Build history of the part. All positions in model axes, mm. Face numbers are marked on the shaded views. A direction names the side the tool comes from. Coordinates: 2 decimals unless noted, no trailing zeros. Loops run counter-clockwise (first coordinate to the right, second up) from the corner with the lowest first, then second, coordinate; pieces in that order, holes last.
Item 1: Drill centre lines: line 1 along Y through (x, z) = (23, 0.6); line 2 along X through (y, z) = (1.25, 0.5); line 3 along Z through (x, y) = (6, 6.5). Where is each one in solid material? Low to high.
Item 2: Cut at B-B (x = 12.5). List the corners of the cut face in (y, z), and give its area (3 significant figures).
Item 3: Cut at A-A (y = 14.5). List the corners of the cut face in (x, z), and give its area (4 significant figures).
Item 4: Flat gauge pins, fed straight in: pin 1 (1.2 mm diameter, centred on y = 21, z = -1.5, fed in from +X); pin 2 (2.5 mm diameter, centred on y = 13.5, z = 4.5, fed in from -X); pin 3 (4 mm diameter, centred on x = 9, y = 5, fed in from +Z). Where does each tip first touch, or does it go through?
Item 5: Cut at D-D (x = 20.75). List the corners of the cut face in (y, z), and give its area (3 significant figures).
Item 6: Cut at C-C (z = -1). List the corners of the cut face in (x, y), and give its area (3 significant figures).
Item 7: 3-axis set-ups, long thin cutter, end or side, ignore diameter. For the marked faces 1, 2, 3 and 4: which of +Z, -Z, +X, -X, +Y, -Y reach the whole face in a straight line?
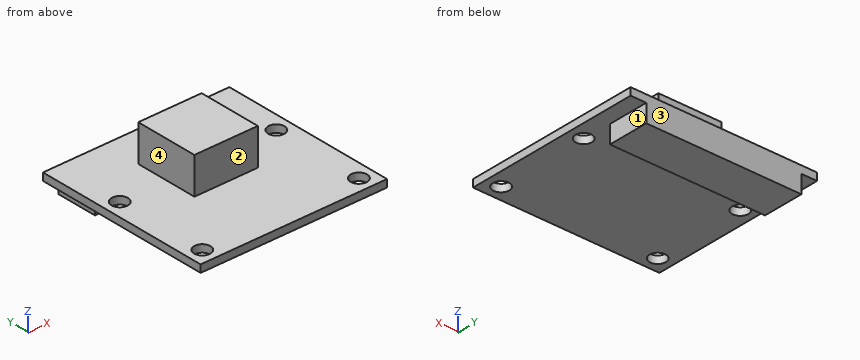
from build123d import *

# Parameters (mm, degrees)
F0_W     = 25
F0_H     = 23.862
F0_R     = 1.1
F1_DEPTH = 1
F2_W     = 20.8
F2_H     = 5.5
F3_DEPTH = 2.4
F4_W     = 8.5
F4_H     = 8.5
F5_DEPTH = 4.9


with BuildPart() as f1:
    # F0 (on Top) → F1 (new body)
    with BuildSketch(Plane.XY):
        with Locations((12.5, 11.931)):
            Rectangle(F0_W, F0_H)
        with Locations((2, 2)):
            Circle(F0_R, mode=Mode.SUBTRACT)
        with Locations((23, 2)):
            Circle(F0_R, mode=Mode.SUBTRACT)
        with Locations((2, 14.5)):
            Circle(F0_R, mode=Mode.SUBTRACT)
        with Locations((23, 14.5)):
            Circle(F0_R, mode=Mode.SUBTRACT)
    extrude(amount=F1_DEPTH)

    # F2 (on face) → F3 (join)
    with BuildSketch(Plane(origin=(0, 0, 0), x_dir=(1, 0, 0), z_dir=(0, 0, -1))):
        with Locations((12.5, -21.112)):
            Rectangle(F2_W, F2_H)
    extrude(amount=F3_DEPTH)

    # F4 (on face) → F5 (join)
    with BuildSketch(Plane.XY.offset(1)):
        with Locations((12.5, 14.5)):
            Rectangle(F4_W, F4_H)
    extrude(amount=F5_DEPTH)


solid = f1.part
Filled sheet:
1. line 1: y = 0 to 0.9, 3.1 to 13.4, 15.6 to 23.86
1. line 2: x = 0 to 1.2, 2.8 to 22.2, 23.8 to 25
1. line 3: z = 0 to 1
2. outline: (0, 0) - (18.36, 0) - (18.36, -2.4) - (23.86, -2.4) - (23.86, 1) - (18.75, 1) - (18.75, 5.9) - (10.25, 5.9) - (10.25, 1) - (0, 1) - close
2. area: 78.7 mm2
3. outline: (0, 0) - (0.9, 0) - (0.9, 1) - (0, 1) - close; (3.1, 0) - (21.9, 0) - (21.9, 1) - (16.75, 1) - (16.75, 5.9) - (8.25, 5.9) - (8.25, 1) - (3.1, 1) - close; (24.1, 0) - (25, 0) - (25, 1) - (24.1, 1) - close
3. area: 62.25 mm2
4. pin 1: stops at x = 22.9
4. pin 2: stops at x = 8.25
4. pin 3: stops at z = 1
5. outline: (0, 0) - (18.36, 0) - (18.36, -2.4) - (23.86, -2.4) - (23.86, 1) - (0, 1) - close
5. area: 37.1 mm2
6. outline: (2.1, 18.36) - (22.9, 18.36) - (22.9, 23.86) - (2.1, 23.86) - close
6. area: 114 mm2
7. face 1: -Z, +X, +Y, -Y
7. face 2: +Z, +X, -X, -Y
7. face 3: +Z, -Z, +X, -X, +Y
7. face 4: +Z, -X, +Y, -Y
